```python
from build123d import *

# Parameters (mm, degrees)
CYLINDER001_R     = 6.45
CYLINDER001_DEPTH = 5
CYLINDER002_R     = 9
CYLINDER002_DEPTH = 5
CHAMFER_SIZE      = 2


with BuildPart() as exterior:
    # Cylinder001 → Cylinder001 (new body)
    with BuildSketch(Plane.XY):
        Circle(CYLINDER001_R)
    extrude(amount=CYLINDER001_DEPTH)


with BuildPart() as cut:
    # Cylinder002 → Cylinder002 (new body)
    with BuildSketch(Plane.XY):
        Circle(CYLINDER002_R)
    extrude(amount=CYLINDER002_DEPTH)

    # Chamfer
    chamfer_edges = [cut.edges().sort_by_distance(p)[0] for p in [
        (-9, 0, 5),
        (-9, 0, 0),
    ]]
    chamfer(chamfer_edges, length=CHAMFER_SIZE)

    # Cut: cut exterior
    add(exterior.part, mode=Mode.SUBTRACT)


solid = cut.part
```
Build history of the part. All positions in model axes, mm. Coordinates: 2 decimals unless noted, no trailing zeros. Order: outer loops, then holes, each group sorted by start corner. A loop starts at its lowest first (then second) coordinate and runs counter-clockwise, first axis right, second up.
Item 1: Saw through at D-D on z = 3.45. List the corners of the cut face in (x, y), then the cut area to 3 significant figures.
Filled in:
outline: circle Ø17.1 at (0, 0); hole circle Ø12.9 at (0, 0)
area: 99.0 mm2
Item 2: Saw through at A-A on x = 0. List the corners of the cut face in (y, z), then the cut area to 3 significant figures.
Filled in:
outline: (-9, 2) - (-7, 0) - (-6.45, 0) - (-6.45, 5) - (-7, 5) - (-9, 3) - close; (6.45, 0) - (7, 0) - (9, 2) - (9, 3) - (7, 5) - (6.45, 5) - close
area: 17.5 mm2
Item 3: Mould opens along Y. For faces 1 (the cylindrical face through (-1.398, -6.297, 2.465)), 2 (the cylindrical face through (-1.172, 8.923, 2.493)), 3 (the flat face through (3, -6, 5)) say: released by +Y, released by -Y, zero draft, split by the parting line, or undercut.
Filled in:
face 1: undercut
face 2: split by the parting line
face 3: zero draft
Item 4: Drill centre lines: L1, parallel to Y at x = 0, z = 2.1; L2, parallel to Y at x = -0.5, z = 0.45; L3, parallel to X at y = 2, z = 0.3. Where is each one in solid material? Low to high.
Filled in:
L1: y = -9 to -6.45, 6.45 to 9
L2: y = -7.43 to -6.43, 6.43 to 7.43
L3: x = -7.02 to -6.13, 6.13 to 7.02
Item 5: Saw through at C-C on z = 0.8. List the corners of the cut face in (x, y), then the cut area to 3 significant figures.
Filled in:
outline: circle Ø15.6 at (0, 0); hole circle Ø12.9 at (0, 0)
area: 60.4 mm2
